```python
from build123d import *

# Parameters (mm, degrees)
SKETCH1_R           = 6
SKETCH1_R_2         = 2.4
BOSS_EXTRUDE1_DEPTH = 8
SKETCH2_R           = 11
SKETCH2_R_2         = 6
BOSS_EXTRUDE2_DEPTH = 10
SKETCH3_R           = 10.75
SKETCH3_R_2         = 6
BOSS_EXTRUDE3_DEPTH = 17


with BuildPart() as part:
    # Sketch1 → Boss-Extrude1 (new body)
    with BuildSketch(Plane(origin=(0, 0, 0), x_dir=(1, 0, 0), z_dir=(0, 1, 0))):
        with BuildLine():
            Line((-15, 14.696938457), (-15, -14.696938457))
            ThreePointArc((-15, -14.696938457), (0, -21), (15, -14.696938457))
            Line((15, -14.696938457), (15, 14.696938457))
            ThreePointArc((15, 14.696938457), (0, 21), (-15, 14.696938457))
        make_face()
        Circle(SKETCH1_R, mode=Mode.SUBTRACT)
        with Locations((0, 16)):
            Circle(SKETCH1_R_2, mode=Mode.SUBTRACT)
        with Locations((11.313708499, 11.313708499)):
            Circle(SKETCH1_R_2, mode=Mode.SUBTRACT)
        with Locations((-11.313708499, 11.313708499)):
            Circle(SKETCH1_R_2, mode=Mode.SUBTRACT)
        with Locations((11.313708499, -11.313708499)):
            Circle(SKETCH1_R_2, mode=Mode.SUBTRACT)
        with Locations((0, -16)):
            Circle(SKETCH1_R_2, mode=Mode.SUBTRACT)
        with Locations((-11.313708499, -11.313708499)):
            Circle(SKETCH1_R_2, mode=Mode.SUBTRACT)
    extrude(amount=BOSS_EXTRUDE1_DEPTH)

    # Sketch2 → Boss-Extrude2 (add)
    with BuildSketch(Plane.XZ):
        Circle(SKETCH2_R)
        Circle(SKETCH2_R_2, mode=Mode.SUBTRACT)
    extrude(amount=BOSS_EXTRUDE2_DEPTH)

    # Sketch3 → Boss-Extrude3 (add)
    with BuildSketch(Plane.XZ.offset(10)):
        Circle(SKETCH3_R)
        Circle(SKETCH3_R_2, mode=Mode.SUBTRACT)
    extrude(amount=BOSS_EXTRUDE3_DEPTH)


solid = part.part
```
For this review, take the finished solid that the model builds, in its own axes (mm). A direction names the side the tool comes from. Coordinates: 2 decimals unless noted, no trailing zeros. Write each loop counter-clockwise with the first axis right and the second up, starting at its lowest first coordinate (ties: lowest second). Pieces come first, ordered by that corner, then holes. Notation, with made-up numbers: (84.5, 64.5) - (97.5, 64.5) arc R27 cw to (97.5, 92.5) - close; hole circle Ø9 at (49.25, -15). An arc over 180 degrees is marked (long way). Put each result on its own line as item: value.
1. For pin 1 (6 mm diameter, centred on x = -11, y = -13.5, fed in from -Z); pin 2 (6 mm diameter, centred on y = -18.5, z = -1, fed in from -X); pin 3 (10 mm diameter, centred on x = 7.5, z = -14.5, fed in from -Y), all flat-tipped, find the tip position at first contact; note any pin that passes through.
Values found:
pin 1: z = -7.18
pin 2: x = -10.75
pin 3: y = 0
2. Machinability: for faces 1 (the flat face through (-7, 0, 9)), 2 (the cylindrical face through (1.29, 3.944, 13.976)), which of the approach directions +Z, -Z, +X, -X, +Y, -Y give a long, thin tool a straight path to every point of the face, cutting with its end or side? Answer none if there is none.
Values found:
face 1: -Y
face 2: +Y, -Y
3. Add section A-A, the plane z = 0. Give the boundary of the cut face in (x, y).
Values found:
outline: (-15, 0) - (-11, 0) - (-11, -10) - (-10.75, -10) - (-10.75, -27) - (-6, -27) - (-6, 8) - (-15, 8) - close; (6, -27) - (10.75, -27) - (10.75, -10) - (11, -10) - (11, 0) - (15, 0) - (15, 8) - (6, 8) - close
4. Add section B-B, the plane x = 0. Give the boundary of the cut face in (y, z).
Values found:
outline: (-27, -10.75) - (-10, -10.75) - (-10, -11) - (0, -11) - (0, -13.6) - (8, -13.6) - (8, -6) - (-27, -6) - close; (-27, 6) - (8, 6) - (8, 13.6) - (0, 13.6) - (0, 11) - (-10, 11) - (-10, 10.75) - (-27, 10.75) - close; (0, -21) - (8, -21) - (8, -18.4) - (0, -18.4) - close; (0, 18.4) - (8, 18.4) - (8, 21) - (0, 21) - close
5. Add section D-D, the plane y = 5. Give the boundary of the cut face in (x, z), then the cut area to 3 significant figures.
Values found:
outline: (-15, -14.7) arc R21 ccw to (15, -14.7) - (15, 14.7) arc R21 ccw to (-15, 14.7) - close; hole circle Ø4.8 at (-11.31, -11.31); hole circle Ø4.8 at (-11.31, 11.31); hole circle Ø12 at (0, 0); hole circle Ø4.8 at (0, -16); hole circle Ø4.8 at (0, 16); hole circle Ø4.8 at (11.31, -11.31); hole circle Ø4.8 at (11.31, 11.31)
area: 921 mm²
6. Add section C-C, the plane x = 5. Give the boundary of the cut face in (y, z).
Values found:
outline: (-27, -9.52) - (-10, -9.52) - (-10, -9.8) - (0, -9.8) - (0, -20.4) - (8, -20.4) - (8, -3.32) - (-27, -3.32) - close; (-27, 3.32) - (8, 3.32) - (8, 20.4) - (0, 20.4) - (0, 9.8) - (-10, 9.8) - (-10, 9.52) - (-27, 9.52) - close
7. Wall thickness on probe 1 along X at (y, z) = (7.5, -13); probe 2 along Z at (x, y) = (-0.5, 0.5); probe 3 along Y at (x, z) = (-7.5, -16.5): over which ranges is each line inside the solid? List them lowest first.
Values found:
probe 1: -15 to -13.02, -9.61 to 9.61, 13.02 to 15
probe 2: -20.99 to -18.35, -13.65 to -5.98, 5.98 to 13.65, 18.35 to 20.99
probe 3: 0 to 8
